from build123d import *

# Parameters (mm, degrees)
BOSS_EXTRUDE2_DEPTH = 5.715
SKETCH2_R           = 3.048
CUT_EXTRUDE1_DEPTH  = 2.8702
FILLET1_R           = 1.27
FILLET2_R           = 1.27
FILLET3_R           = 0.762


with BuildPart() as part:
    # Sketch1 → Boss-Extrude2 (new body)
    with BuildSketch(Plane(origin=(0, 0, 0), x_dir=(1, 0, 0), z_dir=(0, 1, 0))):
        Polygon((-12.7, 15.59701387), (0, 15.59701387), (0, 2.89701387), (12.7, 2.89701387), (12.7, -22.50298613), (0, -22.50298613), (0, -9.80298613), (-12.7, -9.80298613), align=None)
    extrude(amount=BOSS_EXTRUDE2_DEPTH)

    # Sketch2 → Cut-Extrude1 (cut)
    with BuildSketch(Plane(origin=(0, 5.715, 0), x_dir=(1, 0, 0), z_dir=(0, 1, 0))):
        with Locations(Location((-6.35, 9.24701387, 0), (0, 0, 270))):
            Circle(SKETCH2_R)
        with Locations(Location((6.35, -16.15298613, 0), (0, 0, 270))):
            Circle(SKETCH2_R)
        with Locations(Location((-6.35, -3.45298613, 0), (0, 0, 270))):
            Circle(SKETCH2_R)
        with Locations(Location((6.35, -3.45298613, 0), (0, 0, 270))):
            Circle(SKETCH2_R)
    extrude(amount=-CUT_EXTRUDE1_DEPTH, mode=Mode.SUBTRACT)

    # Fillet1
    fillet1_edges = [part.edges().sort_by_distance(p)[0] for p in [
        (-6.35, 5.715, -15.59701387),
        (0, 5.715, -9.24701387),
        (6.35, 5.715, -2.89701387),
        (12.7, 5.715, 9.80298613),
        (6.35, 5.715, 22.50298613),
        (0, 5.715, 16.15298613),
        (-6.35, 5.715, 9.80298613),
        (-12.7, 5.715, -2.89701387),
    ]]
    fillet(fillet1_edges, radius=FILLET1_R)

    # Fillet2
    fillet2_edges = [part.edges().sort_by_distance(p)[0] for p in [
        (-12.7, 0, -2.89701387),
        (-6.35, 0, 9.80298613),
        (0, 0, 16.15298613),
        (6.35, 0, 22.50298613),
        (12.7, 0, 9.80298613),
        (6.35, 0, -2.89701387),
        (0, 0, -9.24701387),
        (-6.35, 0, -15.59701387),
    ]]
    fillet(fillet2_edges, radius=FILLET2_R)

    # Fillet3
    fillet3_edges = [part.edges().sort_by_distance(p)[0] for p in [
        (-6.35, 5.715, -12.29501387),
        (6.35, 5.715, 0.40498613),
        (-6.35, 5.715, 0.40498613),
        (6.35, 5.715, 13.10498613),
    ]]
    fillet(fillet3_edges, radius=FILLET3_R)


solid = part.part
Verification items for the finished model (mm, model axes). A direction names the side the tool comes from. Give positions to 0.01 mm unless a question says otherwise; leave off trailing zeros. Write each loop counter-clockwise with the first axis right and the second up, starting at its lowest first coordinate (ties: lowest second). Pieces come first, ordered by that corner, then holes. Notation, with made-up numbers: M -19.5,20.25 L 34.5,20.25 A24 ccw 34.5,37.25 Z; hole C 40,65 d6. An arc over 180 degrees is marked long. Put each result on its own line as item: value. Start each with the question number.
1. Section check D-D (y = 0.9). Record the cut outline in (x, z), and give its area (3 significant figures).
2. Section check A-A (x = 6.35). Record the cut outline in (y, z) (3 decimals).
3. Draft check along X on faces 1 (the face through (0.38, 5.35, 15.42)), 2 (the face through (-6.216, 3.914, -12.292)), 3 (the face through (0, 0, 3)). Enter one of: +X half, -X half, draft (parallel to the pull), parting line (faces both ways), or undercut.
4. Go/stop test with flat-tipped pins: pin 1 Ø3 at (x, z) = (-7.5, -9.5) entering from +Y; pin 2 Ø1.5 at (y, z) = (3, -4) entering from +X; pin 3 Ø1 at (x, z) = (-5.5, 10.5) entering from -Y; pin 4 Ø2.5 at (x, y) = (9.5, 3) entering from -Z. Record where each tip stops, or that it passes through.
5. Scan lines: line 1 along Z through (x, y) = (7.5, 3.3); line 2 along X through (y, z) = (3.6, 6); line 3 along Z through (x, y) = (6.5, 5.4). Record each from-to range of solid material in increasing order. Write a range as [from, to].
6. Section check C-C (z = -5). Record the cut outline in (x, y) (3 decimals), and give its area (3 significant figures).
7. Set-up check for faces 4 (the face through (-5.813, 5.353, 9.421)), 5 (the face through (-6, 3, 9.803)), 6 (the face through (6, 2.845, 3)), 7 (the face through (-0.382, 0.362, -8.514)): record each of +Z, -Z, +X, -X, +Y, -Y from which the full face is reachable in a straight line by a thin tool's end or side.
8. Section check B-B (y = 3.6). Record the cut outline in (x, z), and give its area (3 significant figures).
Answer list:
1. outline: M -12.64,-15.54 L -0.06,-15.54 L -0.06,-2.84 L 12.64,-2.84 L 12.64,22.45 L 0.06,22.45 L 0.06,9.75 L -12.64,9.75 Z
1. area: 638 mm2
2. outline: M 0,-1.627 A1.27 ccw 1.27,-2.897 L 4.445,-2.897 A1.27 ccw 5.715,-1.627 L 5.715,-0.357 A0.762 ccw 4.953,0.405 L 2.845,0.405 L 2.845,6.501 L 4.953,6.501 A0.762 ccw 5.715,7.263 L 5.715,12.343 A0.762 ccw 4.953,13.105 L 2.845,13.105 L 2.845,19.201 L 4.953,19.201 A0.762 ccw 5.715,19.963 L 5.715,21.233 A1.27 ccw 4.445,22.503 L 1.27,22.503 A1.27 ccw 0,21.233 Z
3. face 1: -X half
3. face 2: undercut
3. face 3: draft
4. pin 1: y = 2.84
4. pin 2: x = 0
4. pin 3: through
4. pin 4: z = -2.9
5. line 1: [-2.9, 0.63], [6.28, 13.33], [18.98, 22.5]
5. line 2: [-12.7, -8.02], [-4.68, 4.68], [8.02, 12.7]
5. line 3: [-2.46, 0.26], [6.64, 12.96], [19.34, 22.07]
6. outline: M -12.7,1.27 A1.27 ccw -11.43,0 L -1.27,0 A1.27 ccw 0,1.27 L 0,4.445 A1.27 ccw -1.27,5.715 L -11.43,5.715 A1.27 ccw -12.7,4.445 Z
6. area: 71.2 mm2
7. face 4: +Z, -X, +Y
7. face 5: +Z, -X, +Y, -Y
7. face 6: +Y
7. face 7: -Z, +X, -Y
8. outline: M -12.7,-15.6 L 0,-15.6 L 0,-2.9 L 12.7,-2.9 L 12.7,22.5 L 0,22.5 L 0,9.8 L -12.7,9.8 Z; hole C -6.35,-9.25 d6.1; hole C -6.35,3.45 d6.1; hole C 6.35,3.45 d6.1; hole C 6.35,16.15 d6.1
8. area: 528 mm2
